```python
from build123d import *

# Parameters (mm, degrees)
SKETCH1_R           = 39.6875
SKETCH1_R_2         = 19.84375
BOSS_EXTRUDE1_DEPTH = 158.75
SKETCH2_R           = 79.375
BOSS_EXTRUDE2_DEPTH = 158.75


with BuildPart() as part:
    # Sketch1 → Boss-Extrude1 (new body)
    with BuildSketch(Plane(origin=(0, 0, 0), x_dir=(1, 0, 0), z_dir=(0, 1, 0))):
        Polygon((158.75, -79.375), (79.375, -238.125), (-79.375, -238.125), (-158.75, -79.375), (-158.75, 79.375), (-105.833333333, 79.375), (-79.375, 132.291666667), (0, 132.291666667), (79.375, 132.291666667), (105.833333333, 79.375), (158.75, 79.375), align=None)
        with Locations(Location((-99.21875, 0, 0), (0, 0, 90))):
            Circle(SKETCH1_R, mode=Mode.SUBTRACT)
        with Locations(Location((99.21875, 0, 0), (0, 0, 90))):
            Circle(SKETCH1_R, mode=Mode.SUBTRACT)
        with Locations(Location((-59.53125, 105.833333333, 0), (0, 0, 90))):
            Circle(SKETCH1_R_2, mode=Mode.SUBTRACT)
        with Locations(Location((59.53125, 105.833333333, 0), (0, 0, 90))):
            Circle(SKETCH1_R_2, mode=Mode.SUBTRACT)
    extrude(amount=BOSS_EXTRUDE1_DEPTH)

    # Sketch2 → Boss-Extrude2 (add)
    with BuildSketch(Plane.XY.offset(238.125)):
        with Locations((0, 4.842306375)):
            Circle(SKETCH2_R)
    extrude(amount=BOSS_EXTRUDE2_DEPTH)


solid = part.part
```
For this review, take the finished solid that the model builds, in its own axes (mm). A direction names the side the tool comes from. Round coordinates to 2 decimals unless told otherwise and drop trailing zeros. Write each loop counter-clockwise with the first axis right and the second up, starting at its lowest first coordinate (ties: lowest second). Pieces come first, ordered by that corner, then holes. Notation, with made-up numbers: (36, 43) - (90, 43) arc R25 ccw to (90, 70) - close; hole circle Ø7 at (-8.5, 81.5). An arc over 180 degrees is marked (long way). Write each question's results on one line, items separated by ' | '.
Item 1: To check wall thickness, follow line 1 along X through (y, z) = (46, 0); line 2 along Y through (x, z) = (-132.5, 124); line 3 along Z through (x, y) = (51, 144.5) (3 decimals). State the ranges of each line that lie inside material, in increasing order. Write a range as from..to.
Calculated:
line 1: x = -158.75..-138.91, -59.53..59.53, 138.91..158.75 | line 2: y = 0..158.75 | line 3: z = -132.292..-123.75, -87.917..238.125
Item 2: Draft analysis for pull direction Z (two halves, no side actions). For faces 5 (the face through (132, 78, -79.375)), 6 (the face through (-158.75, 78, 1)), 7 (the face through (-79.206, 78.264, -103.25)), state which applies: pulls with the +Z half, pulls with the -Z half, needs draft (parallel to the pull), parting line crosses it, or undercut.
Calculated:
face 5: pulls with the -Z half | face 6: needs draft | face 7: undercut
Item 3: For faces 1 (the face through (-17.207, -72.645, 316.389)), 2 (the face through (-138.57, 78.26, 5.17)), 3 (the face through (-133, 78, -79.375)), 4 (the face through (-1, -28, 238.125)), list the 3-axis set-ups (+Z, -Z, +X, -X, +Y, -Y) from which the entire face can be reached by the end or side of a thin tool; tool diameter is ignored.
Calculated:
face 1: +Z | face 2: +Y, -Y | face 3: -Z, -X, +Y, -Y | face 4: -Z, +X, -X, -Y
Item 4: For pin 1 (8 mm diameter, centred on x = 59.5, z = 39.5, fed in from -Y); pin 2 (16 mm diameter, centred on x = 129, y = 88, fed in from -Z) (3 decimals); pin 3 (8 mm diameter, centred on x = 73.5, z = 330.5, fed in from -Y), all flat-tipped, find the tip position at first contact; note any pin that passes through.
Calculated:
pin 1: stops at y = 0 | pin 2: stops at z = -79.375 | pin 3: stops at y = -33.5
Item 5: Take a section at C-C on y = 73.5. Count the separate pieces of the cut face and the enclosed holes in it, then the cut area to 3 significant figures.
Calculated:
separate pieces: 1 | enclosed holes: 4 | area: 98,300 mm^2
Item 6: Take a section at D-D on x = 0. State the section outline as (y, z) points (3 decimals).
Calculated:
outline: (-74.533, 238.125) - (0, 238.125) - (0, -132.292) - (158.75, -132.292) - (158.75, 238.125) - (84.217, 238.125) - (84.217, 396.875) - (-74.533, 396.875) - close
Item 7: Take a section at B-B on x = -46.5. State the section outline as (y, z) points (3 decimals), then the cut area to 3 significant figures.
Calculated:
outline: (-59.486, 238.125) - (0, 238.125) - (0, -90.868) - (158.75, -90.868) - (158.75, 238.125) - (69.171, 238.125) - (69.171, 396.875) - (-59.486, 396.875) - close; (0, -132.292) - (158.75, -132.292) - (158.75, -120.799) - (0, -120.799) - close | area: 74,500 mm^2
Item 8: Take a section at A-A on z = 0. State the section outline as (x, y) points.
Calculated:
outline: (-158.75, 0) - (-138.91, 0) - (-138.91, 158.75) - (-158.75, 158.75) - close; (-59.53, 0) - (59.53, 0) - (59.53, 158.75) - (-59.53, 158.75) - close; (138.91, 0) - (158.75, 0) - (158.75, 158.75) - (138.91, 158.75) - close
